Here's how the part is built. I have some questions about the finished solid (model axes, mm). A direction names the side the tool comes from. Coordinates: 2 decimals unless noted, no trailing zeros. Write each loop counter-clockwise with the first axis right and the second up, starting at its lowest first coordinate (ties: lowest second). Pieces come first, ordered by that corner, then holes. Notation, with made-up numbers: M 83.25,43 L 93.25,43 A14 ccw 93.25,67 Z; hole C -39.5,5 d10. An arc over 180 degrees is marked long. Use one line per item in the form item = value. Start each with the question number.
1. I want a section at C-C, the plane z = -331. List the corners of the cut face in (x, y) for me, plus the area to 3 significant figures.
2. I want a section at D-D, the plane y = -138.5. List the corners of the cut face in (x, z) for me, plus the area to 3 significant figures.
3. Thinking about a two-plate mould opening in Y: for faces 6 (the face through (43.752, 31.742, 12.522)), 7 (the face through (-3, -127, -636)), 8 (the face through (-17, 50.8, -587)), 9 (the face through (76.2, -25, 13)), which applies, released by +Y, released by -Y, zero draft, split by the parting line, or undercut?
4. Please list where these lines run through material, in increasing order: line 1 along Z through (x, y) = (181.5, 40.5); line 2 along X through (y, z) = (-59, -477); line 3 along Z through (x, y) = (-96.5, 13.5). Write a range as [from, to].
5. I want a section at B-B, the plane x = 44.45. List the corners of the cut face in (y, z) for me.
6. I'm going to push flat-ended pins straight in: pin 1 Ø8 at (y, z) = (-92, -175.5) entering from +X; pin 2 Ø15 at (x, z) = (-175.5, 17) entering from -Y; pin 3 Ø8 at (x, y) = (-48, -81) entering from +Z; pin 4 Ø20.5 at (x, y) = (27.5, -138.5) entering from +Z. Where does each tip first touch, or does it pass through?
7. I want a section at A-A, the plane z = -659.5. List the corners of the cut face in (x, y) for me, plus the area to 3 significant figures.
8. On a 3-axis mill with a long thin cutter (end or side, diameter ignored), from which of +Z, -Z, +X, -X, +Y, -Y can I reach the whole of each face in a straight line? I mean faces 1 (the face through (-89, -50.8, 13)), 2 (the face through (-3, -140, -584.2)), 3 (the face through (3, 12, 25.4)), 4 (the face through (-196.67, -100.89, -275.13)), 5 (the face through (-3, 38, -584.2)). Say none if no direction works.
from build123d import *

# Parameters (mm, degrees)
F1_DEPTH = 25.4
F3_DEPTH = 25.4
F5_W     = 25.4
F5_H     = 101.6
F6_DEPTH = 368.3
F7_W     = 419.1
F7_H     = 203.2
F8_DEPTH = 25.4


with BuildPart() as f1:
    # F0 (on Top) → F1 (new body)
    with BuildSketch(Plane.XY):
        with BuildLine():
            Line((184.15, -50.8), (184.15, 50.8))
            Line((184.15, 50.8), (-184.15, 50.8))
            Line((-184.15, 50.8), (-184.15, -50.8))
            Line((-184.15, -50.8), (-165.1, -50.8))
            Line((-165.1, -50.8), (-165.1, 0))
            ThreePointArc((-165.1, 0), (-133.35, 31.75), (-101.6, 0))
            Line((-101.6, 0), (-101.6, -50.8))
            Line((-101.6, -50.8), (-76.2, -50.8))
            Line((-76.2, -50.8), (-76.2, 0))
            ThreePointArc((-76.2, 0), (-44.45, 31.75), (-12.7, 0))
            Line((-12.7, 0), (-12.7, -50.8))
            Line((-12.7, -50.8), (12.7, -50.8))
            Line((12.7, -50.8), (12.7, 0))
            ThreePointArc((12.7, 0), (44.45, 31.75), (76.2, 0))
            Line((76.2, 0), (76.2, -50.8))
            Line((76.2, -50.8), (101.6, -50.8))
            Line((101.6, -50.8), (101.6, 0))
            ThreePointArc((101.6, 0), (133.35, 31.75), (165.1, 0))
            Line((165.1, 0), (165.1, -50.8))
            Line((165.1, -50.8), (184.15, -50.8))
        make_face()
    extrude(amount=F1_DEPTH)

    # F2 (on face) → F3 (join)
    with BuildSketch(Plane.YZ.offset(184.15)):
        Polygon((50.8, -685.8), (50.8, 25.4), (-50.8, 25.4), (-152.4, -584.2), (-152.4, -685.8), align=None)
    extrude(amount=F3_DEPTH)

    # F4: F1 across plane


with BuildPart() as f1_1:
    add(f1.part)
    add(f1.part.mirror(Plane.YZ))

    # F5 (on face) → F6 (join, through all)
    with BuildSketch(Plane.YZ.offset(-184.15)):
        with Locations((-139.7, -635)):
            Rectangle(F5_W, F5_H)
        with Locations((38.1, -635)):
            Rectangle(F5_W, F5_H)
    extrude(amount=F6_DEPTH)

    # F7 (on face) → F8 (join)
    with BuildSketch(Plane(origin=(0, 0, -685.8), x_dir=(1, 0, 0), z_dir=(0, 0, -1))):
        with Locations((0, 50.8)):
            Rectangle(F7_W, F7_H)
    extrude(amount=F8_DEPTH)


solid = f1_1.part
Answer list:
q1.outline = M -209.55,-110.2 L -184.15,-110.2 L -184.15,50.8 L -209.55,50.8 Z; M 184.15,-110.2 L 209.55,-110.2 L 209.55,50.8 L 184.15,50.8 Z
q1.area = 8,180 mm²
q2.outline = M -209.55,-711.2 L 209.55,-711.2 L 209.55,-500.8 L 184.15,-500.8 L 184.15,-584.2 L -184.15,-584.2 L -184.15,-500.8 L -209.55,-500.8 Z
q2.area = 57,500 mm²
q3.face_6 = released by -Y
q3.face_7 = undercut
q3.face_8 = released by +Y
q3.face_9 = zero draft
q4.line_1 = [-711.2, -584.2], [0, 25.4]
q4.line_2 = [-209.55, -184.15], [184.15, 209.55]
q4.line_3 = [-711.2, -685.8], [0, 25.4]
q5.outline = M -152.4,-711.2 L 50.8,-711.2 L 50.8,-584.2 L 25.4,-584.2 L 25.4,-685.8 L -127,-685.8 L -127,-584.2 L -152.4,-584.2 Z; M 31.75,0 L 50.8,0 L 50.8,25.4 L 31.75,25.4 Z
q6.pin_1 = through
q6.pin_2 = -50.8
q6.pin_3 = -685.8
q6.pin_4 = -584.2
q7.outline = M -209.55,-152.4 L 209.55,-152.4 L 209.55,50.8 L -209.55,50.8 Z; hole M -184.15,-127 L 184.15,-127 L 184.15,25.4 L -184.15,25.4 Z
q7.area = 29,000 mm²
q8.face_1 = +Z, -Y
q8.face_2 = +Z, +Y, -Y
q8.face_3 = +Z, +X, -X, +Y, -Y
q8.face_4 = +Z, +X, -X, -Y
q8.face_5 = +Y, -Y
